Here's how the part is built. I have some questions about the finished solid (model axes, mm). A direction names the side the tool comes from. Round coordinates to 2 decimals unless told otherwise and drop trailing zeros. Write each loop counter-clockwise with the first axis right and the second up, starting at its lowest first coordinate (ties: lowest second). Pieces come first, ordered by that corner, then holes. Notation, with made-up numbers: (-19.5, 32) - (31.5, 32) arc R36 ccw to (31.5, 71) - close; hole circle Ø4 at (4, 29). An arc over 180 degrees is marked (long way). Use one line per item in the form item = value. Start each with the question number.
1. I want a section at D-D, the plane z = -4.5. List the corners of the cut face in (x, y) for me.
2. If I drill on line 1 along Z through (x, y) = (-18.5, 9); line 2 along X through (y, z) = (6.25, -15); line 3 along X through (y, z) = (5, 13), over which ranges is the centre line in solid material (lowest first)?
3. I want a section at B-B, the plane x = 12.5. List the corners of the cut face in (y, z) for me.
4. I want a section at C-C, the plane y = 3. List the corners of the cut face in (x, z) for me, plus the area to 3 significant figures.
5. We'd pull the mould along Y, two halves only. Please class faces 1 (the flat face through (0, 0, 0)), 2 (the flat face through (0, 6, -35)), 3 (the cylindrical face through (16.89, 5.38, 23.03)): +Y half, -Y half, draft (parallel to the pull), parting line (faces both ways), or undercut.
6. Will these pins go through, and if not, where does the flat tip stop? pin 1 (2.5 mm diameter, centred on y = 6, z = 25, fed in from -X); pin 2 (3.5 mm diameter, centred on y = 6, z = -25, fed in from +X); pin 3 (3.5 mm diameter, centred on x = -18.5, z = -15, fed in from +Y).
7. I want a section at A-A, the plane z = -15. List the corners of the cut face in (x, y) for me.
8. Which directions (+Z, -Z, +X, -X, +Y, -Y) give clear straight access to the entire face, cutting with the end or side of a thin tool? Please do faces 4 (the flat face through (-15, 12, 0)), 5 (the cylindrical face through (16.893, 4.563, 0.211)), 6 (the flat face through (-2, 9, 0)), 7 (the cylindrical face through (-16.89, 5.38, -23.03)).
Autodesk Inventor part; units mm, degrees
ref_plane "YZ Plane" through (0, 0, 0) normal (1, 0, 0) x (0, 1, 0)
ref_plane "XZ Plane" through (0, 0, 0) normal (0, 1, 0) x (-1, 0, 0)
ref_plane "XY Plane" through (0, 0, 0) normal (0, 0, 1) x (1, 0, 0)
sketch "Skizze_Grundkörper" plane through (0, 0, 0) normal (0, 0, 1) x (1, 0, 0)
  line L0 (-25, 0) -> (25, 0)
  line L1 (25, 0) -> (25, 12)
  line L2 (25, 12) -> (5, 12)
  line L3 (-35, 0) -> (35, 0)
  line L4 (0, -2.4) -> (0, 14.4)
  line L5 (5, 12) -> (0, 7)
  line L6 (0, 7) -> (-5, 12)
  line L7 (-5, 12) -> (-25, 12)
  line L8 (-25, 12) -> (-25, 0)
  point P0 (0, 0)
  dimension "Breite" = 50
  dimension "Höhe" = 12
  dimension "Nuttiefe" = 5
  dimension "Nutwinkel" = 90
extrude "Grundkörper" add sketch "Skizze_Grundkörper" along normal mid plane 70
sketch "Skizze_Bohrung_6H7" plane through (-25, 12, 35) normal (0, 1, 0) x (1, 0, 0)
  line L0 (-10, 35) -> (60, 35)
  line L1 (25, 84) -> (25, -14)
  point P0 (25, 35)
  point P1 (6.5, 50)
  point P2 (43.5, 50)
  point P3 (43.5, 20)
  point P4 (6.5, 20)
  dimension "Abstand_Breite_Bohrung_6H7" = 37
  dimension "Abstand_Länge_Bohrung_6H7" = 30
hole "Bohrung_6H7" at (-18.5, 12, -15) at (18.5, 12, -15) at (18.5, 12, 15) at (-18.5, 12, 15) direction (0, -1, 0) diameter 6 end through all
sketch "Skizze_Gewinde_M4" plane through (-25, 0, 35) normal (0, -1, 0) x (1, 0, 0)
  line L0 (-10, -35) -> (60, -35)
  line L1 (25, -84) -> (25, 14)
  point P0 (25, -35)
  point P1 (6.5, -35)
  point P2 (43.5, -35)
  dimension "Abstand_Breite_Gewinde_M4" = 37
hole "Gewinde_M4" at (-18.5, 0, 0) at (18.5, 0, 0) direction (0, 1, 0) diameter 3.242 depth 9 tip angle 118
sketch "Skizze_Gewinde_M5" plane through (25, 0, 35) normal (1, 0, 0) x (0, 0, -1)
  line L0 (35, -2.4) -> (35, 14.4)
  line L1 (84, 0) -> (-14, 0)
  point P0 (35, 0)
  point P1 (10, 6)
  point P2 (60, 6)
  dimension "Abstand_Länge_Gewinde_M5" = 50
  dimension "Abstand_Höhe_Gewinde_M5" = 6
hole "Gewinde_M5" at (25, 6, 25) at (25, 6, -25) direction (-1, 0, 0) diameter 4.134 depth 16 tip angle 118
pattern_circular "Anordnung_Gewinde_M5" count 2 over 360 about axis through (0, -10, 0) along (0, 1, 0) of "Gewinde_M5"
properties part number "Unterstempel_2016_iLogic"
Model answer:
q1.outline = (-25, 0) - (25, 0) - (25, 12) - (5, 12) - (0, 7) - (-5, 12) - (-25, 12) - close
q2.line_1 = -35 to -18, -12 to -1.62, 1.62 to 12, 18 to 35
q2.line_2 = -25 to -21.5, -15.5 to 15.5, 21.5 to 25
q2.line_3 = -25 to -20.74, -16.26 to 16.26, 20.74 to 25
q3.outline = (0, -35) - (12, -35) - (12, 35) - (0, 35) - close; hole circle Ø4.13 at (6, -25); hole circle Ø4.13 at (6, 25)
q4.outline = (-25, -35) - (25, -35) - (25, 35) - (-25, 35) - close; hole circle Ø6 at (-18.5, -15); hole circle Ø6 at (-18.5, 15); hole circle Ø3.24 at (-18.5, 0); hole circle Ø6 at (18.5, -15); hole circle Ø6 at (18.5, 15); hole circle Ø3.24 at (18.5, 0)
q4.area = 3,370 mm2
q5.face_1 = -Y half
q5.face_2 = draft
q5.face_3 = undercut
q6.pin_1 = -8.51
q6.pin_2 = 8.81
q6.pin_3 = through
q7.outline = (-25, 0) - (-21.5, 0) - (-21.5, 12) - (-25, 12) - close; (-15.5, 0) - (15.5, 0) - (15.5, 12) - (5, 12) - (0, 7) - (-5, 12) - (-15.5, 12) - close; (21.5, 0) - (25, 0) - (25, 12) - (21.5, 12) - close
q8.face_4 = +Z, -Z, +X, -X, +Y
q8.face_5 = -Y
q8.face_6 = +Z, -Z, +Y
q8.face_7 = -X
